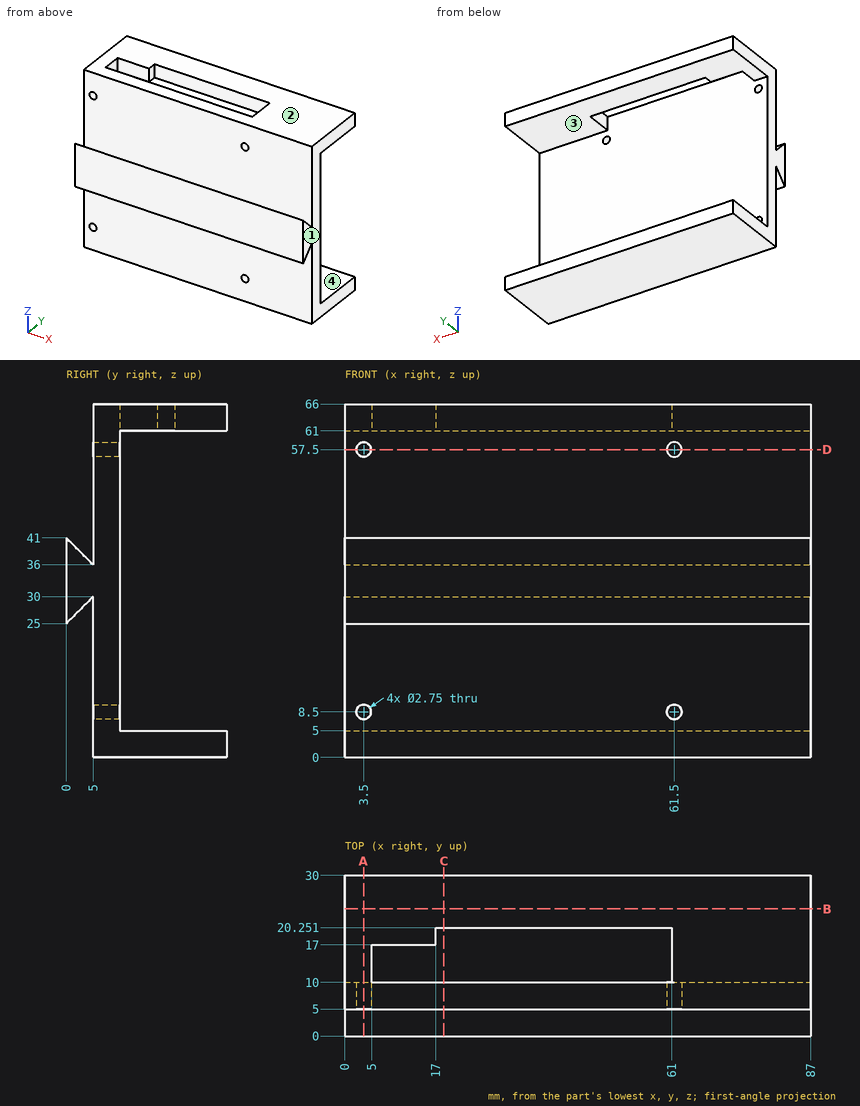
Verification items for this drawing (mm, ordinates from the low corner). Give positions to 0.01 mm unless a question says otherwise; leave off trailing zeros. Write each loop counter-clockwise with the first axis right and the second up, starting at its lowest first coordinate (ties: lowest second). Pieces come first, ordered by that corner, then holes. Notation, with made-up numbers: (49.5, 15.5) - (100.5, 15.5) arc R25 ccw to (100.5, 29.5) - close; hole circle Ø2 at (-37.75, 35). An arc over 180 degrees is marked (long way). Answer as a JSON object with one key per item and string values. Group by question number.
1) Thickness scan on probe 1 along Z at (x, y) = (61.5, 7.2) (1 decimal); probe 2 along X at (y, z) = (7.45, 57.5) (1 decimal); probe 3 along Z at (x, y) = (18, 28.5). Record the ranges inside material, lowest first. Write a range as from..to.
2) Sectioned sample at C-C (x = 18.5). Record the cut outline in (y, z).
3) Sectioned sample at A-A (x = 3.5). Record the cut outline in (y, z) (1 decimal).
4) Sectioned sample at D-D (z = 57.5). Record the cut outline in (x, y) (1 decimal).
5) Release check for a two-part mould opening along Z. For the marked faces 1, 2, 3 and 4 record: pulls with the +Z half, pulls with the -Z half, needs draft (parallel to the pull), parting line crosses it, or undercut.
6) Sectioned sample at B-B (y = 23.75). Record the cut outline in (x, z).
7) Depth check by flat-ended pin: P1, Ø24, axis at x = 59.5, z = 8, coming from the -Y side; P2, Ø1.6, axis at x = 61.5, z = 57.5, coming from the -Y side; P3, Ø12, axis at x = 58.5, z = 48.5, coming from the +Y side. Enter the tip coordinate at first touch or a pass-through.
Geometry results:
{
 "1": {"probe 1": "z = 0..7.1, 9.9..56.1, 58.9..66", "probe 2": "x = 0..2.1, 4.9..60.1, 62.9..87", "probe 3": "z = 0..5, 61..66"},
 "2": {"outline": "(0, 25) - (5, 30) - (5, 0) - (30, 0) - (30, 5) - (10, 5) - (10, 66) - (5, 66) - (5, 36) - (0, 41) - close; (20.25, 61) - (30, 61) - (30, 66) - (20.25, 66) - close"},
 "3": {"outline": "(0, 25) - (5, 30) - (5, 9.9) - (10, 9.9) - (10, 56.1) - (5, 56.1) - (5, 36) - (0, 41) - close; (5, 0) - (30, 0) - (30, 5) - (10, 5) - (10, 7.1) - (5, 7.1) - close; (5, 58.9) - (10, 58.9) - (10, 61) - (30, 61) - (30, 66) - (5, 66) - close"},
 "4": {"outline": "(0, 5) - (2.1, 5) - (2.1, 10) - (0, 10) - close; (4.9, 5) - (60.1, 5) - (60.1, 10) - (4.9, 10) - close; (62.9, 5) - (87, 5) - (87, 10) - (62.9, 10) - close"},
 "5": {"face 1": "needs draft", "face 2": "pulls with the +Z half", "face 3": "undercut", "face 4": "undercut"},
 "6": {"outline": "(0, 0) - (87, 0) - (87, 5) - (0, 5) - close; (0, 61) - (87, 61) - (87, 66) - (0, 66) - close"},
 "7": {"P1": "stops at y = 5", "P2": "passes through", "P3": "stops at y = 10"}
}
